```python
from build123d import *

# Parameters (mm, degrees)
REVOLUTION002_ANGLE = 160
PAD003_DEPTH        = 35
FILLET_R            = 10
SKETCH016_R         = 2.1
POCKET006_DEPTH     = 34.2030828023


with BuildPart() as part:
    # Sketch013 → Revolution002 (revolve, symmetric)
    with BuildSketch(Plane.XZ) as revolution002_sk:
        with BuildLine():
            Line((-14.592572, -91.29162), (-14.592572, -78.10162))
            ThreePointArc((-14.592572, -78.10162), (-14.8782194915, -77.2178434814), (-15.6270897945, -76.6684358973))
            Line((-15.6270897945, -76.6684358973), (-19.0629351267, -75.5285381595))
            ThreePointArc((-19.8645151397, -74.4180577621), (-19.6431856264, -75.1028382434), (-19.0629351267, -75.5285381595))
            Line((-19.8645151397, -74.4180577621), (-19.8645151397, -73.7280577621))
            ThreePointArc((-19.1361680024, -72.7285381595), (-19.6631126608, -73.1096871232), (-19.8645151397, -73.7280577621))
            Line((-19.1361680024, -72.7285381595), (-15.100012655, -71.4296732661))
            ThreePointArc((-15.100012655, -71.4296732661), (-14.5676210475, -71.009067316), (-14.4410938084, -70.3424782022))
            Line((-14.4410938084, -70.3424782022), (-14.6116789932, -69.3469880241))
            ThreePointArc((-14.6116789932, -69.3469880241), (-15.0652099201, -68.5548455589), (-15.922572, -68.24162))
            Line((-15.922572, -68.24162), (-27.932572, -68.24162))
            ThreePointArc((-27.932572, -68.24162), (-29.1487956636, -68.7453963364), (-29.652572, -69.96162))
            Line((-29.652572, -69.96162), (-29.652572, -91.29162))
            Line((-29.652572, -91.29162), (-14.592572, -91.29162))
        make_face()
    revolve(axis=Axis((0, 0, 0), (0, 0, 1)), revolution_arc=REVOLUTION002_ANGLE / 2)
    revolve(revolution002_sk.sketch, axis=Axis((0, 0, 0), (0, 0, -1)), revolution_arc=REVOLUTION002_ANGLE / 2)

    # Sketch014 (on Face8 of Revolution002) → Pad003 (new body)
    with BuildSketch(Plane(origin=(0, 0, -91.29162), x_dir=(1, 0, 0), z_dir=(0, 0, -1))):
        with BuildLine():
            Line((-29.2279836153, 5), (-13.7092362141, 5))
            ThreePointArc((-13.7092362141, 5), (-14.592572, 0), (-13.7092362141, -5))
            Line((-29.2279836153, -5), (-13.7092362141, -5))
            ThreePointArc((-29.2279836153, 5), (-29.652572, 0), (-29.2279836153, -5))
        make_face()
    extrude(amount=PAD003_DEPTH)

    # Fillet
    fillet_edges = [part.edges().sort_by_distance(p)[0] for p in [
        (-29.652572, 0, -126.29162),
    ]]
    fillet(fillet_edges, radius=FILLET_R)

    # Sketch016 (on Face2 of Fillet) → Pocket006 (cut, through all)
    with BuildSketch(Plane.XZ.offset(5)):
        with Locations((-19.005882937, -116.29162)):
            Circle(SKETCH016_R)
    extrude(amount=-POCKET006_DEPTH, mode=Mode.SUBTRACT)


solid = part.part
```
Input: part model. Units: mm. Frame: model coordinates. A direction names the side the tool comes from. Coordinates: 2 decimals unless noted, no trailing zeros. Loops run counter-clockwise (first coordinate to the right, second up) from the corner with the lowest first, then second, coordinate; pieces in that order, holes last. Notation, with made-up numbers: M -13.5,12 L 33.5,12 A21 cw 33.5,49 Z; hole C 9.5,-27 d11. An arc over 180 degrees is marked long. Answer in a Markdown table with one row per item.
1. Reachability of faces 4 (the flat face through (-16, 15, -91.292)), 5 (the flat face through (-22, -5, -109)), 6 (the conical face through (-15.839, -0.31, -76.597)), 7 (the flat face through (-18, 0, -68.242)) from +Z, -Z, +X, -X, +Y, -Y: full face, straight path, thin tool, end or side. Return the list, or none.
Response:
| item | result |
|---|---|
| face 4 | -Z, +X, -X, +Y |
| face 5 | -Z, +X, -X, -Y |
| face 6 | +X |
| face 7 | +Z, +X, -X, +Y, -Y |
2. First-contact query: pin 1 (5 mm diameter, centred on x = -19.01, z = -116.29, fed in from +Y); pin 2 (12 mm diameter, centred on x = -22.5, y = -22.5, fed in from -Z); pin 3 (3 mm diameter, centred on x = -11, z = -112, fed in from +Y); pin 4 (8 mm diameter, centred on y = -6, z = -101.5, fed in from +X). Flat tips, straight axial feed; report the tip coordinate or a pass-through.
Response:
| item | result |
|---|---|
| pin 1 | stops at y = 5 |
| pin 2 | stops at z = -91.29 |
| pin 3 | passes through |
| pin 4 | stops at x = -13.71 |
3. Draft query along X for faces 1 (the flat face through (-3.846, -21.81, -79.605)), 2 (the flat face through (-16, -17, -91.292)), 3 (the cylindrical face through (-19.46, -0.07, -118.34)). Return one class per face: pulls with the +X half, pulls with the -X half, needs draft (parallel to the pull), parting line crosses it, or undercut.
Response:
| item | result |
|---|---|
| face 1 | pulls with the +X half |
| face 2 | needs draft |
| face 3 | undercut |
4. Section C-C, the plane z = -96.5. Output: boundary loops of the cut face in (x, y), then the cut area to 3 significant figures.
Response:
| item | result |
|---|---|
| outline | M -29.23,-5 L -13.71,-5 A14.59 cw -13.71,5 L -29.23,5 A29.65 ccw Z |
| area | 152 mm2 |
5. Section B-B, the plane z = -87.5. Output: boundary loops of the cut face in (x, y).
Response:
| item | result |
|---|---|
| outline | M -5.15,-29.2 L -2.53,-14.37 A14.59 cw -2.53,14.37 L -5.15,29.2 A29.65 ccw Z |
6. Section A-A, the plane y = 0. Output: boundary loops of the cut face in (x, z).
Response:
| item | result |
|---|---|
| outline | M -29.65,-116.29 A10 ccw -19.65,-126.29 L -14.59,-126.29 L -14.59,-78.1 A1.51 ccw -15.63,-76.67 L -19.06,-75.53 A1.17 cw -19.86,-74.42 L -19.86,-73.73 A1.05 cw -19.14,-72.73 L -15.1,-71.43 A0.97 ccw -14.44,-70.34 L -14.61,-69.35 A1.33 ccw -15.92,-68.24 L -27.93,-68.24 A1.72 ccw -29.65,-69.96 Z; hole C -19.01,-116.29 d4.2 |
7. Material intervals for line 1 (Y direction, x = -16, z = -111); line 2 (Y direction, x = -8, z = -80.5); line 3 (Z direction, x = -13.5, y = 14), sorted ascending.
Response:
| item | result |
|---|---|
| line 1 | y = -5 to 5 |
| line 2 | y = -28.55 to -12.2, 12.2 to 28.55 |
| line 3 | z = -91.29 to -75.31, -72.89 to -68.24 |
